```python
from build123d import *

# Parameters (mm, degrees)
BOSS_EXTRUDE1_DEPTH = 3.175
FILLET1_R           = 12.7


with BuildPart() as part:
    # Sketch2 → Boss-Extrude1 (new body)
    with BuildSketch(Plane(origin=(0, 631.882105473, 103.848248331), x_dir=(1, 0, 0), z_dir=(0, 0.9867625124381899, 0.16217195826243017))):
        Polygon((100, -1224.067157157), (100, -1137.347457675), (154.094451659, -1137.347457675), (162.370253897, -969.61100369), (100, -969.61100369), (100, -954.242157057), (48.689491118, -954.242157057), (53.570568791, -855.31100369), (-53.570568791, -855.31100369), (-48.689491118, -954.242157057), (-100, -954.242157057), (-109.652, -954.242157057), (-109.652, -969.61100369), (-162.370253897, -969.61100369), (-154.094451659, -1137.347457675), (-109.652, -1137.347457675), (-109.652, -1224.067157157), (-100, -1224.067157157), (-35.376831367, -1224.067157157), (-34.016071035, -1251.647457675), (34.016071035, -1251.647457675), (35.376831367, -1224.067157157), align=None)
    extrude(amount=-BOSS_EXTRUDE1_DEPTH)

    # Fillet1
    fillet1_edges = [part.edges().sort_by_distance(p)[0] for p in [
        (34.016071035, 427.333500719, 1338.66959037),
        (-34.016071035, 427.333500719, 1338.66959037),
        (-154.094451659, 445.869755548, 1225.882635198),
        (-162.370253897, 473.071904763, 1060.366590436),
        (-53.570568791, 491.608159593, 947.579635264),
        (53.570568791, 491.608159593, 947.579635264),
        (162.370253897, 473.071904763, 1060.366590436),
        (154.094451659, 445.869755548, 1225.882635198),
    ]]
    fillet(fillet1_edges, radius=FILLET1_R)


solid = part.part
```
Geometry: final body of the model. Coordinates: model frame, mm. A direction names the side the tool comes from. Coordinates: 2 decimals unless noted, no trailing zeros. Order: outer loops, then holes, each group sorted by start corner. A loop starts at its lowest first (then second) coordinate and runs counter-clockwise, first axis right, second up. Notation, with made-up numbers: (60.25, -34.75) -> (107.25, -34.75) arc R22 ccw to (107.25, -12.75) -> close; hole circle Ø7 at (75, -5.75). An arc over 180 degrees is marked (long way). Write each question's results on one line, items separated by ' | '. Start each with the question number.
1) Material intervals for line 1 along Y through (x, z) = (-103.5, 1295.5); line 2 along Y through (x, z) = (57.5, 1216.5); line 3 along X through (y, z) = (430, 1322), sorted ascending.
2) Mould query, pull axis X, two halves, no side actions, for faces 3 (the flat face through (100, 439, 1269)), 4 (the cylindrical face through (-30.8, 427.9, 1335.1)), 5 (the flat face through (-2.264, 458.354, 1140.13)). Classes: released by +X, released by -X, zero draft, split by the parting line, or undercut.
3) Set-up query: faces 1 (the flat face through (-2.264, 461.487, 1140.644)), 2 (the flat face through (-109.652, 439, 1268)). Return all of +Z, -Z, +X, -X, +Y, -Y with unobstructed straight access to the full face (end or side cutting, diameter ignored); none if empty.
4) Cut plane A-A, the plane x = 5. Output: boundary loops of the cut face in (y, z).
5) First-contact query: pin 1 (4.5 mm diameter, centred on y = 475, z = 1049, fed in from +X); pin 2 (3 mm diameter, centred on x = 24, z = 1224, fed in from +Y); pin 3 (10 mm diameter, centred on x = 79, z = 1235.5, fed in from +Y). Flat tips, straight axial feed; report the tip coordinate or a pass-through.
6) Cut plane B-B, the plane z = 994. Output: boundary loops of the cut face in (x, y).
Checks:
1) line 1: 432.82 to 436.04 | line 2: 445.8 to 449.02 | line 3: -34.85 to 34.85
2) face 3: released by +X | face 4: released by -X | face 5: zero draft
3) face 1: +Z, +X, -X, +Y | face 2: +Z, -X, +Y, -Y
4) outline: (425.77, 1338.41) -> (490.04, 947.32) -> (493.17, 947.84) -> (428.9, 1338.93) -> close
5) pin 1: x = 100 | pin 2: y = 448.03 | pin 3: y = 446.72
6) outline: (-51.26, 485.59) -> (-51.24, 482.37) -> (51.24, 482.37) -> (51.26, 485.59) -> close
